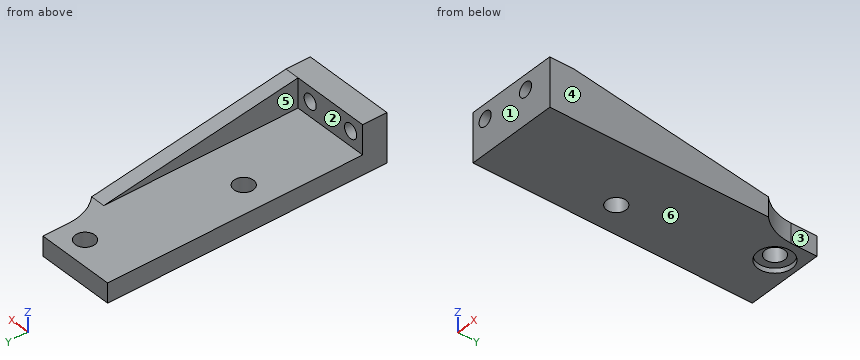
from build123d import *

# Parameters (mm, degrees)
SKETCH_1_W          = 16
SKETCH_1_H          = 6
SKETCH_1_R          = 1.5
EXTRUDE_1_DEPTH     = 5
SKETCH_2_W          = 16
SKETCH_2_H          = 57.5
EXTRUDE_2_DEPTH     = 4
SKETCH_3_R          = 2
CUT_EXTRUDE_1_DEPTH = 60.213596412
SKETCH_4_R          = 2
CUT_EXTRUDE_2_DEPTH = 60.213596412
SKETCH_5_R          = 3.5
CUT_EXTRUDE_3_DEPTH = 1
EXTRUDE_3_DEPTH     = 3
FILLET_1_R          = 10


with BuildPart() as part:
    # 草图1 → 凸台-拉伸1 (new body)
    with BuildSketch(Plane(origin=(0, 0, 0), x_dir=(1, 0, 0), z_dir=(0, 1, 0))):
        with Locations((2, 0)):
            Rectangle(SKETCH_1_W, SKETCH_1_H)
        with Locations(Location((-3, 0, 0), (0, 0, 270))):
            Circle(SKETCH_1_R, mode=Mode.SUBTRACT)
        with Locations(Location((7, 0, 0), (0, 0, 270))):
            Circle(SKETCH_1_R, mode=Mode.SUBTRACT)
    extrude(amount=EXTRUDE_1_DEPTH)

    # 草图2 → 凸台-拉伸2 (add)
    with BuildSketch(Plane(origin=(0, 0, -3), x_dir=(-1, 0, 0), z_dir=(0, 0, -1))):
        with Locations((-2, 28.75)):
            Rectangle(SKETCH_2_W, SKETCH_2_H)
    extrude(amount=EXTRUDE_2_DEPTH)

    # 草图3 → 切除-拉伸1 (cut, through all)
    with BuildSketch(Plane(origin=(0, 0, -7), x_dir=(-1, 0, 0), z_dir=(0, 0, -1))):
        with Locations((-5, 53)):
            Circle(SKETCH_3_R)
    extrude(amount=-CUT_EXTRUDE_1_DEPTH, mode=Mode.SUBTRACT)

    # 草图4 → 切除-拉伸2 (cut, through all)
    with BuildSketch(Plane(origin=(0, 0, -7), x_dir=(-1, 0, 0), z_dir=(0, 0, -1))):
        with Locations((0, 24.5)):
            Circle(SKETCH_4_R)
    extrude(amount=-CUT_EXTRUDE_2_DEPTH, mode=Mode.SUBTRACT)

    # 草图5 → 切除-拉伸3 (cut)
    with BuildSketch(Plane(origin=(0, 0, -7), x_dir=(-1, 0, 0), z_dir=(0, 0, -1))):
        with Locations((-5, 53)):
            Circle(SKETCH_5_R)
    extrude(amount=-CUT_EXTRUDE_3_DEPTH, mode=Mode.SUBTRACT)

    # 草图6 → 凸台-拉伸3 (add)
    with BuildSketch(Plane(origin=(10, 0, 0), x_dir=(0, 0, -1), z_dir=(1, 0, 0))):
        Polygon((3, 45), (3, 5), (-3, 5), (-3, 0), (7, 0), (7, 45), align=None)
        Polygon((-3, 5), (3, 5), (3, 45), align=None)
    extrude(amount=EXTRUDE_3_DEPTH)

    # 圆角1
    # the kernel refuses this fillet: 10 mm, written as the material it adds along each edge
    with BuildSketch(Plane(origin=(10, 45, -7), x_dir=(0, 1, 0), z_dir=(0, 0, 1))) as fillet_1_piece_1:
        with BuildLine():
            CenterArc((7.141428429, -10), FILLET_1_R, 90, 45.572995999)
            Line((0, -3), (0, 0))
            Line((0, 0), (7.141428429, 0))
        make_face()
    extrude(amount=4)


solid = part.part
Read the model definition and answer for the solid it produces. Units are mm, in the model's axes. Face numbers are marked on the shaded views. A direction names the side the tool comes from. Coordinates: 2 decimals unless noted, no trailing zeros. Order: outer loops, then holes, each group sorted by start corner. A loop starts at its lowest first (then second) coordinate and runs counter-clockwise, first axis right, second up. Notation, with made-up numbers: M 27,80.25 L 62,80.25 A30 ccw 62,106.25 Z; hole C 50,70 d1. An arc over 180 degrees is marked long. Put each result on its own line as item: value. Start each with the question number.
Item 1: Section A-A, the plane x = 0 is taken. Determine the outline of the cut face in (y, z), plus the area to 3 significant figures.
Item 2: The mould has two halves that part along X. Classify the marked faces 4, 5 and 6: +X half, -X half, draft (parallel to the pull), parting line (faces both ways), or undercut.
Item 3: Section D-D, the plane x = -3 is taken. Determine the outline of the cut face in (y, z).
Item 4: Consider probe 1 along X at (y, z) = (2, 0); probe 2 along Y at (x, z) = (5, -6.35); probe 3 along Y at (x, z) = (0, -5.55). Determine where each line is inside the solid, lowest interval first. Write a range as [from, to].
Item 5: Given pin 1 Ø3 at (x, y) = (5, 53) entering from -Z; pin 2 Ø1.2 at (y, z) = (55.5, -6) entering from +X; pin 3 Ø8 at (x, y) = (5, 53) entering from +Z; pin 4 Ø2 at (x, y) = (3.5, 52) entering from -Z, each flat-ended and moving along its own axis, determine where each tip first touches the part or whether it passes through.
Item 6: Section C-C, the plane y = 4.5 is taken. Determine the outline of the cut face in (x, z).
Item 7: Section B-B, the plane y = 53 is taken. Determine the outline of the cut face in (x, z), plus the area to 3 significant figures.
Item 8: For the marked faces 1, 2 and 3, determine the directions among +Z, -Z, +X, -X, +Y, -Y from which every point of the face is accessible in a straight line to the end or side of a thin tool.
Computed:
1. outline: M 0,-7 L 22.5,-7 L 22.5,-3 L 5,-3 L 5,3 L 0,3 Z; M 26.5,-7 L 57.5,-7 L 57.5,-3 L 26.5,-3 Z
1. area: 244 mm2
2. face 4: +X half
2. face 5: -X half
2. face 6: draft
3. outline: M 0,-7 L 57.5,-7 L 57.5,-3 L 5,-3 L 5,-1.5 L 0,-1.5 Z; M 0,1.5 L 5,1.5 L 5,3 L 0,3 Z
4. probe 1: x = [-6, -4.5], [-1.5, 5.5], [8.5, 13]
4. probe 2: y = [0, 49.5], [56.5, 57.5]
4. probe 3: y = [0, 22.5], [26.5, 57.5]
5. pin 1: passes through
5. pin 2: stops at x = 10
5. pin 3: stops at z = -3
5. pin 4: stops at z = -6
6. outline: M -6,-7 L 13,-7 L 13,3 L -6,3 Z; hole C -3,0 d3; hole C 7,0 d3
7. outline: M -6,-7 L 1.5,-7 L 1.5,-6 L 3,-6 L 3,-3 L -6,-3 Z; M 7,-6 L 8.5,-6 L 8.5,-7 L 10,-7 L 10,-3 L 7,-3 Z
7. area: 45.0 mm2
8. face 1: +Z, -Z, +X, -X, -Y
8. face 2: +Z, -X, +Y
8. face 3: +Z, -Z, +X, +Y
